Verification items for the finished model (mm, model axes). Face numbers are marked on the shaded views. A direction names the side the tool comes from. Give positions to 0.01 mm unless a question says otherwise; leave off trailing zeros. Loops run counter-clockwise (first coordinate to the right, second up) from the corner with the lowest first, then second, coordinate; pieces in that order, holes last. Notation, with made-up numbers: (17.25, 44) - (37.25, 44) arc R20 ccw to (37.25, 73) - close; hole circle Ø9 at (-5, 20). An arc over 180 degrees is marked (long way). One line per question, with ' | ' between items. Start each with the question number.
1. Section check B-B, the plane y = -12. State how many separate pieces and enclosed holes the cut face has, then the cut area to 3 significant figures.
2. Tool access check on the marked faces 4 and 5. Record the directions out of +Z, -Z, +X, -X, +Y, -Y that give a thin tool (end or side, any length) a straight path to the whole face; none if there is none.
3. Depth check by flat-ended pin: pin 1 Ø5.5 at (x, y) = (38.95, 12) entering from -Z. Enter the tip coordinate at first touch or a pass-through.
4. Section check A-A, the plane x = 14.65. Enter the section's corners in (y, z).
5. Thickness scan on line 1 along Y through (x, z) = (22, 8); line 2 along Y through (x, z) = (30.85, 1.15); line 3 along X through (y, z) = (-10, 9.75). Record the ranges inside material, lowest first. Write a range as from..to.
6. Section check D-D, the plane x = -3. Enter the section's corners in (y, z), then the cut area to 3 significant figures.
7. Mould release check, pull along Y, two halves, no side actions. Record for the marked faces 1, 2 and 3: +Y half, -Y half, draft (parallel to the pull), parting line (faces both ways), or undercut.
from build123d import *

# Parameters (mm, degrees)
F0_W     = 95
F0_H     = 40
F1_DEPTH = 14.6
F2_W     = 88.9
F2_H     = 10
F3_DEPTH = 12.6
F4_W     = 1
F4_H     = 1.5
F5_DEPTH = 12.6
F6_R     = 3.5
F7_DEPTH = 14.601
F8_R     = 2
F9_R     = 0.49999


# Not quite as in the source:
# - a fillet or chamfer is up to 0.001 mm smaller than in the source, because OpenCascade refuses the exact size


with BuildPart() as f1:
    # F0 (on Top) → F1 (new body)
    with BuildSketch(Plane.XY):
        Rectangle(F0_W, F0_H)
    extrude(amount=F1_DEPTH)

    # F2 (on face) → F3 (cut)
    with BuildSketch(Plane.XY.offset(14.6)):
        with Locations((0, 12)):
            Rectangle(F2_W, F2_H)
        Rectangle(F2_W, F2_H)
        with Locations((0, -12)):
            Rectangle(F2_W, F2_H)
    extrude(amount=-F3_DEPTH, mode=Mode.SUBTRACT)

    # F4 (on face) → F5 (join, through all)
    with BuildSketch(Plane.XY.offset(14.6)):
        with Locations((-17.95, 16.25)):
            Rectangle(F4_W, F4_H)
        with Locations((8.65, 16.25)):
            Rectangle(F4_W, F4_H)
        with Locations((8.65, 7.75)):
            Rectangle(F4_W, F4_H)
        with Locations((-17.95, 7.75)):
            Rectangle(F4_W, F4_H)
        with Locations((-17.95, 4.25)):
            Rectangle(F4_W, F4_H)
        with Locations((8.65, 4.25)):
            Rectangle(F4_W, F4_H)
        with Locations((8.65, -16.25)):
            Rectangle(F4_W, F4_H)
        with Locations((-17.95, -16.25)):
            Rectangle(F4_W, F4_H)
        with Locations((-17.95, -4.25)):
            Rectangle(F4_W, F4_H)
        with Locations((-17.95, -7.75)):
            Rectangle(F4_W, F4_H)
        with Locations((8.65, -4.25)):
            Rectangle(F4_W, F4_H)
        with Locations((8.65, -7.75)):
            Rectangle(F4_W, F4_H)
    extrude(amount=-F5_DEPTH)

    # F6 (on face) → F7 (cut, through all)
    with BuildSketch(Plane.XY.offset(14.6)):
        with Locations((-39.55, 12)):
            Circle(F6_R)
        with Locations((-31.45, 12)):
            Circle(F6_R)
        with Locations((-23.35, 12)):
            Circle(F6_R)
        with Locations((-12.55, 12)):
            Circle(F6_R)
        with Locations((-4.45, 12)):
            Circle(F6_R)
        with Locations((3.65, 12)):
            Circle(F6_R)
        with Locations((14.65, 12)):
            Circle(F6_R)
        with Locations((22.75, 12)):
            Circle(F6_R)
        with Locations((30.85, 12)):
            Circle(F6_R)
        with Locations((38.95, 12)):
            Circle(F6_R)
        with Locations((-39.55, 0)):
            Circle(F6_R)
        with Locations((-31.45, 0)):
            Circle(F6_R)
        with Locations((-23.35, 0)):
            Circle(F6_R)
        with Locations((-12.55, 0)):
            Circle(F6_R)
        with Locations((-4.45, 0)):
            Circle(F6_R)
        with Locations((3.65, 0)):
            Circle(F6_R)
        with Locations((14.65, 0)):
            Circle(F6_R)
        with Locations((22.75, 0)):
            Circle(F6_R)
        with Locations((30.85, 0)):
            Circle(F6_R)
        with Locations((38.95, 0)):
            Circle(F6_R)
        with Locations((-39.55, -12)):
            Circle(F6_R)
        with Locations((-31.45, -12)):
            Circle(F6_R)
        with Locations((-23.35, -12)):
            Circle(F6_R)
        with Locations((-12.55, -12)):
            Circle(F6_R)
        with Locations((-4.45, -12)):
            Circle(F6_R)
        with Locations((3.65, -12)):
            Circle(F6_R)
        with Locations((14.65, -12)):
            Circle(F6_R)
        with Locations((22.75, -12)):
            Circle(F6_R)
        with Locations((30.85, -12)):
            Circle(F6_R)
        with Locations((38.95, -12)):
            Circle(F6_R)
    extrude(amount=-F7_DEPTH, mode=Mode.SUBTRACT)

    # F8
    f8_edges = [f1.edges().sort_by_distance(p)[0] for p in [
        (-47.5, -20, 7.3),
        (47.5, -20, 7.3),
        (47.5, 20, 7.3),
        (-47.5, 20, 7.3),
    ]]
    fillet(f8_edges, radius=F8_R)

    # F9 (radius 0.5 in the source; OpenCascade refuses exactly that, so slightly less here)
    f9_edges = [f1.edges().sort_by_distance(p)[0] for p in [
        (-18.45, 17, 8.3),
        (-18.45, 15.5, 8.3),
        (-17.45, 15.5, 8.3),
        (8.15, 17, 8.3),
        (8.15, 15.5, 8.3),
        (9.15, 15.5, 8.3),
        (8.15, 8.5, 8.3),
        (-18.45, 8.5, 8.3),
        (-18.45, 5, 8.3),
        (-18.45, 3.5, 8.3),
        (-17.45, 3.5, 8.3),
        (8.15, 5, 8.3),
        (8.15, 3.5, 8.3),
        (-18.45, -3.5, 8.3),
        (8.15, -3.5, 8.3),
        (-18.45, -8.5, 8.3),
        (-17.45, -8.5, 8.3),
        (-18.45, -7, 8.3),
        (8.15, -7, 8.3),
        (8.15, -8.5, 8.3),
        (9.15, -8.5, 8.3),
        (8.15, -15.5, 8.3),
        (-18.45, -15.5, 8.3),
        (-17.45, -17, 8.3),
        (-17.45, -15.5, 8.3),
        (9.15, -17, 8.3),
        (9.15, -15.5, 8.3),
        (9.15, -5, 8.3),
        (9.15, -3.5, 8.3),
        (9.15, 8.5, 8.3),
        (9.15, 3.5, 8.3),
        (-17.45, -3.5, 8.3),
        (-17.45, -5, 8.3),
        (-17.45, 8.5, 8.3),
        (-17.45, 7, 8.3),
        (9.15, 7, 8.3),
        (8.15, -17, 8.3),
        (-18.45, -17, 8.3),
        (-18.45, -5, 8.3),
        (-18.45, 7, 8.3),
        (8.15, 7, 8.3),
        (9.15, -7, 8.3),
        (9.15, 5, 8.3),
        (-17.45, 5, 8.3),
        (-17.45, -7, 8.3),
        (9.15, 17, 8.3),
        (-17.45, 17, 8.3),
    ]]
    fillet(f9_edges, radius=F9_R)


solid = f1.part
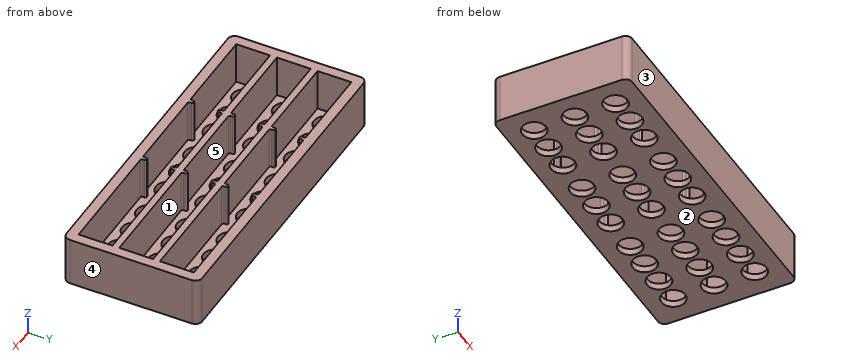
Results list:
1) separate pieces: 11 | enclosed holes: 0 | area: 127 mm²
2) face 4: +Z, -Z, +X, +Y, -Y | face 5: +Z
3) pin 1: through
4) outline: (-20, 0) - (-15.5, 0) - (-15.5, 2) - (-17, 2) - (-17, 14.6) - (-20, 14.6) - close; (-8.5, 0) - (-3.5, 0) - (-3.5, 2) - (-5, 2) - (-5, 14.6) - (-7, 14.6) - (-7, 2) - (-8.5, 2) - close; (3.5, 0) - (8.5, 0) - (8.5, 2) - (7, 2) - (7, 14.6) - (5, 14.6) - (5, 2) - (3.5, 2) - close; (15.5, 0) - (20, 0) - (20, 14.6) - (17, 14.6) - (17, 2) - (15.5, 2) - close
5) line 1: -20..-17, -7..-5, 5..7, 17..20 | line 2: -20..-15.5, -8.5..-3.5, 3.5..8.5, 15.5..20 | line 3: -47.5..-44.45, 44.45..47.5
6) outline: (-20, 0) - (-15.19, 0) - (-15.19, 2) - (-17, 2) - (-17, 14.6) - (-20, 14.6) - close; (-8.81, 0) - (-3.19, 0) - (-3.19, 2) - (-5, 2) - (-5, 14.6) - (-7, 14.6) - (-7, 2) - (-8.81, 2) - close; (3.19, 0) - (8.81, 0) - (8.81, 2) - (7, 2) - (7, 14.6) - (5, 14.6) - (5, 2) - (3.19, 2) - close; (15.19, 0) - (20, 0) - (20, 14.6) - (17, 14.6) - (17, 2) - (15.19, 2) - close | area: 168 mm²
7) face 1: undercut | face 2: draft | face 3: -Y half
